Design review of the part built by this model. Coordinates are the model's own, in mm. Give positions to 0.01 mm unless a question says otherwise; leave off trailing zeros. Write each loop counter-clockwise with the first axis right and the second up, starting at its lowest first coordinate (ties: lowest second). Pieces come first, ordered by that corner, then holes.
```python
from build123d import *

# Parameters (mm, degrees)
F1_DEPTH = 50.8
F4_DEPTH = 12.7
F4_TAPER = -8
F6_DEPTH = 12.7
F6_TAPER = -10


with BuildPart() as f1:
    # F0 (on Right) → F1 (new body)
    with BuildSketch(Plane.YZ):
        Polygon((-140.8138120502, 0.6983735914), (-138.6619785664, -24.6103129146), (140.7380214336, -24.6103129146), (140.7380214336, 49.6335022594), align=None)
    extrude(amount=F1_DEPTH)

    # F3 (on face) → F4 (cut)
    with BuildSketch(Plane(origin=(0, -4.2468228402, 24.4344050926), x_dir=(1, 0, 0), z_dir=(0, -0.1712378928, 0.9852297113))):
        Polygon((33.9139047941, 117.6632965604), (33.9139047941, 88.0739117662), (50.8, 93.7783047557), (50.8, 112.0805814862), align=None)
        Polygon((50.8, -6.458433345), (50.8, 14.1357549945), (38.8870903277, 18.8930730025), (38.8870903277, -10.6963117917), align=None)
    extrude(amount=-F4_DEPTH, taper=F4_TAPER, mode=Mode.SUBTRACT)

    # F5 (on face) → F6 (cut)
    with BuildSketch(Plane(origin=(0, -4.2468228402, 24.4344050926), x_dir=(1, 0, 0), z_dir=(0, -0.1712378928, 0.9852297113))):
        Polygon((37.663642931, -112.632855773), (50.8, -106.7069470882), (50.8, -92.0567885041), (37.663642931, -85.9662666917), align=None)
    extrude(amount=-F6_DEPTH, taper=F6_TAPER, mode=Mode.SUBTRACT)


solid = f1.part
```
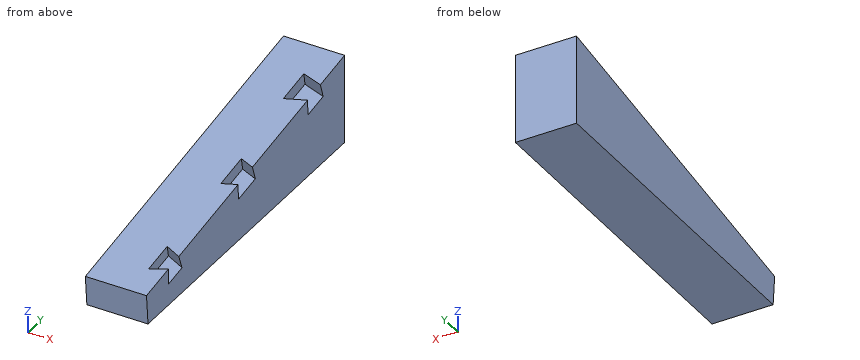
(1) Consider section A-A, the plane x = 18.5. Give the boundary of the cut face in (y, z).
Resolved:
outline: (-140.81, 0.7) - (-138.66, -24.61) - (140.74, -24.61) - (140.74, 49.63) - close
(2) To check wall thickness, follow L1, parallel to Y at x = 13.5, z = 0; L2, parallel to Z at x = 15.5, y = -40; L3, parallel to Z at x = 46, y = -73.5. State the ranges of each line that lie inside material, in increasing order.
Resolved:
L1: y = -140.75 to 140.74
L2: z = -24.61 to 18.22
L3: z = -24.61 to 12.4
(3) Clearance check with flat-ended pins moving along their axes: P1, Ø12, axis at x = 15, y = 37, coming from the +Z side; P2, Ø12, axis at y = 83.5, z = 24.5, coming from the -X side; P3, Ø10, axis at x = 19.5, y = -88, coming from the +Z side. State where each tip first meets the part, or that it passes through.
Resolved:
P1: stops at z = 32.65
P2: stops at x = 0
P3: stops at z = 10.75
(4) Consider section B-B, the plane y = -57. Give the boundary of the cut face in (x, z), then the cut area to 3 significant figures.
Resolved:
outline: (0, -24.61) - (50.8, -24.61) - (50.8, 15.27) - (0, 15.27) - close
area: 2,030 mm2
